Build history of the part. All positions in model axes, mm. A direction names the side the tool comes from. Give positions to 0.01 mm unless a question says otherwise; leave off trailing zeros. Write each loop counter-clockwise with the first axis right and the second up, starting at its lowest first coordinate (ties: lowest second). Pieces come first, ordered by that corner, then holes.
from build123d import *

# Parameters (mm, degrees)
SKETCH4_W                 = 32
SKETCH4_H                 = 35
BOSS_EXTRUDE1_DEPTH       = 9
SHELL1_T                  = -1.5
SHELL1_THICKNESS_2_FACE_W = 29
SHELL1_THICKNESS_2_FACE_H = 32
SHELL1_THICKNESS_2_DEPTH  = 3.4
SKETCH5_R                 = 1.5
CUT_EXTRUDE2_DEPTH        = 9
RIB6_REACH                = 27.362
SKETCH12_WALLS_W          = 81.724747412
SKETCH12_WALLS_H          = 15
SKETCH13_W                = 28
SKETCH13_H                = 8
CUT_EXTRUDE3_DEPTH        = 5
SKETCH15_W                = 24.5
SKETCH15_H                = 2.2
CUT_EXTRUDE4_DEPTH        = 10
SKETCH16_W                = 32
SKETCH16_H                = 4
BOSS_EXTRUDE2_DEPTH       = 9
SKETCH17_W                = 24
SKETCH17_H                = 2.2
CUT_EXTRUDE5_DEPTH        = 10


with BuildPart() as part:
    # Sketch4 → Boss-Extrude1 (new body)
    with BuildSketch(Plane.XY):
        Rectangle(SKETCH4_W, SKETCH4_H)
    extrude(amount=BOSS_EXTRUDE1_DEPTH)

    # Shell1
    shell1_openings = [part.faces().sort_by_distance(p)[0] for p in [
        (0, 0, 9),
    ]]
    offset(amount=SHELL1_T, openings=shell1_openings, kind=Kind.INTERSECTION)

    # Shell1 thickness 2 face (on inner face of the shell) → Shell1 thickness 2 (add)
    with BuildSketch(Plane(origin=(0, 0, 1.5), x_dir=(-1, 0, 0), z_dir=(0, 0, -1))):
        Rectangle(SHELL1_THICKNESS_2_FACE_W, SHELL1_THICKNESS_2_FACE_H)
    extrude(amount=-SHELL1_THICKNESS_2_DEPTH)

    # Sketch5 → Cut-Extrude2 (cut)
    with BuildSketch(Plane.XY.offset(4.9)):
        with Locations((-10, -12)):
            Circle(SKETCH5_R)
        with Locations((10, -12)):
            Circle(SKETCH5_R)
        with Locations((0, 11.7)):
            Circle(SKETCH5_R)
        with Locations((0, -11.7)):
            Circle(SKETCH5_R)
        with Locations((-10, 12)):
            Circle(SKETCH5_R)
        with Locations((10, 12)):
            Circle(SKETCH5_R)
    extrude(amount=-CUT_EXTRUDE2_DEPTH, mode=Mode.SUBTRACT)

    # Sketch12 walls → Rib6 (add, up to next)
    with BuildSketch(Plane.XY.offset(9), mode=Mode.PRIVATE) as rib6_sk1:
        Rectangle(SKETCH12_WALLS_W, SKETCH12_WALLS_H)
    rib6_tool1 = extrude(rib6_sk1.sketch, amount=-RIB6_REACH, mode=Mode.PRIVATE) - part.part
    add(rib6_tool1.solids().sort_by_distance((0, 0, 9))[0])

    # Sketch13 → Cut-Extrude3 (cut)
    with BuildSketch(Plane(origin=(0, 0, 0), x_dir=(-1, 0, 0), z_dir=(0, 0, -1))):
        with Locations((0, -3)):
            Rectangle(SKETCH13_W, SKETCH13_H)
    extrude(amount=-CUT_EXTRUDE3_DEPTH, mode=Mode.SUBTRACT)

    # Sketch15 → Cut-Extrude4 (cut)
    with BuildSketch(Plane(origin=(0, 0, 5), x_dir=(-1, 0, 0), z_dir=(0, 0, -1))):
        with Locations((0.25, -3)):
            Rectangle(SKETCH15_W, SKETCH15_H)
    extrude(amount=-CUT_EXTRUDE4_DEPTH, mode=Mode.SUBTRACT)

    # Sketch16 → Boss-Extrude2 (add)
    with BuildSketch(Plane.XZ.offset(17.5)):
        with Locations((0, 7)):
            Rectangle(SKETCH16_W, SKETCH16_H)
    extrude(amount=BOSS_EXTRUDE2_DEPTH)

    # Sketch17 → Cut-Extrude5 (cut)
    with BuildSketch(Plane.XY.offset(9)):
        with Locations((0, -23.38)):
            Rectangle(SKETCH17_W, SKETCH17_H)
    extrude(amount=-CUT_EXTRUDE5_DEPTH, mode=Mode.SUBTRACT)


solid = part.part
1. Saw through at A-A on x = 3. Give the cut face in (y, z), plus the area to 3 significant figures.
2. Drill centre lines: line 1 along Y through (x, z) = (-10.5, 5.75); line 2 along Y through (x, z) = (0, 4.5); line 3 along Y through (x, z) = (10, 1.75). Where is each one in solid material? Low to high.
3. Mould opens along Y. For faces 4 (the face through (-14.5, -12, 7)), 5 (the face through (16, -4, 4)) say: pulls with the +Y half, pulls with the -Y half, needs draft (parallel to the pull), parting line crosses it, or undercut.
4. Saw through at C-C on z = 7.5. Give the cut face in (x, y), plus the area to 3 significant figures.
5. Drop flat-ended pins along their axis: pin 1 (6.5 mm diameter, centred on x = -5.5, y = -1.5, fed in from -Z); pin 2 (3 mm diameter, centred on x = -7, y = -20, fed in from -Z); pin 3 (2.5 mm diameter, centred on x = 0, y = -11.7, fed in from -Z). Give the stop position or say it passes through.
6. 3-axis set-ups, long thin cutter, end or side, ignore diameter. For faces 1 (the face through (0, -16, 7)), 2 (the face through (12, -3, 7)), 3 (the face through (0, -22, 5)): which of +Z, -Z, +X, -X, +Y, -Y reach the whole face in a straight line?
7. Saw through at B-B on y = -23. Give the cut face in (x, z), plus the area to 3 significant figures.
8. Saw through at D-D on z = 2.5. Give the cut face in (x, y), plus the area to 3 significant figures.
Outcome:
1. outline: (-26.5, 5) - (-24.48, 5) - (-24.48, 9) - (-26.5, 9) - close; (-22.28, 5) - (-17.5, 5) - (-17.5, 0) - (-7, 0) - (-7, 5) - (-4.1, 5) - (-4.1, 9) - (-7.5, 9) - (-7.5, 4.9) - (-16, 4.9) - (-16, 9) - (-22.28, 9) - close; (-1.9, 5) - (1, 5) - (1, 0) - (17.5, 0) - (17.5, 9) - (16, 9) - (16, 4.9) - (7.5, 4.9) - (7.5, 9) - (-1.9, 9) - close
1. area: 224 mm2
2. line 1: y = -26.5 to -24.48, -22.28 to -16, -7.5 to -4.1, -1.9 to 7.5, 16 to 17.5
2. line 2: y = -17.5 to -13.2, -10.2 to -7, 1 to 10.2, 13.2 to 17.5
2. line 3: y = -17.5 to -13.5, -10.5 to -7, 1 to 10.5, 13.5 to 17.5
3. face 4: undercut
3. face 5: needs draft
4. outline: (-16, -26.5) - (16, -26.5) - (16, 17.5) - (-16, 17.5) - close; hole (-14.5, -16) - (14.5, -16) - (14.5, -7.5) - (-14.5, -7.5) - close; hole (-14.5, 7.5) - (14.5, 7.5) - (14.5, 16) - (-14.5, 16) - close; hole (-12.5, -4.1) - (12, -4.1) - (12, -1.9) - (-12.5, -1.9) - close; hole (-12, -24.48) - (12, -24.48) - (12, -22.28) - (-12, -22.28) - close
4. area: 808 mm2
5. pin 1: stops at z = 0
5. pin 2: stops at z = 5
5. pin 3: passes through
6. face 1: +Z
6. face 2: +Z, -Z
6. face 3: -Z, +X, -X, -Y
7. outline: (-16, 5) - (-12, 5) - (-12, 9) - (-16, 9) - close; (12, 5) - (16, 5) - (16, 9) - (12, 9) - close
7. area: 32.0 mm2
8. outline: (-16, -17.5) - (16, -17.5) - (16, 17.5) - (-16, 17.5) - close; hole (-14, -7) - (14, -7) - (14, 1) - (-14, 1) - close; hole circle Ø3 at (-10, -12); hole circle Ø3 at (-10, 12); hole circle Ø3 at (0, -11.7); hole circle Ø3 at (0, 11.7); hole circle Ø3 at (10, -12); hole circle Ø3 at (10, 12)
8. area: 854 mm2
